```python
from build123d import *

# Parameters (mm, degrees)
SKETCH1_R           = 2.3
SKETCH1_R_2         = 4
BOSS_EXTRUDE1_DEPTH = 22.25
FILLET1_R           = 1
FILLET2_R           = 0.5


with BuildPart() as part:
    # Sketch1 → Boss-Extrude1 (new body)
    # profile 1 of 4: a face of its own
    with BuildSketch(Plane(origin=(0, 0, 0), x_dir=(1, 0, 0), z_dir=(0, 1, 0))):
        with BuildLine():
            ThreePointArc((4, 25.4), (0, 21.4), (-4, 25.4))
            Line((-4, 25.4), (-4, 0))
            ThreePointArc((-4, 0), (0, 4), (4, 0))
            ThreePointArc((4, 0), (3.526698395, -1.887431702), (2.218800785, -3.328201177))
            Line((2.218800785, -3.328201177), (40.318800785, 22.071798823))
            ThreePointArc((40.318800785, 22.071798823), (34.271631894, 24.240863405), (38.1, 29.4))
            Line((38.1, 29.4), (0, 29.4))
            ThreePointArc((0, 29.4), (2.828427125, 28.228427125), (4, 25.4))
        make_face()
        Polygon((4, 5.070367517), (4, 21.4), (28.494448725, 21.4), align=None, mode=Mode.SUBTRACT)
        with Locations(Location((12.7, 25.4, 0), (0, 0, 270))):
            Circle(SKETCH1_R, mode=Mode.SUBTRACT)
    # profile 2 of 4: a face of its own
    with BuildSketch(Plane(origin=(0, 0, 0), x_dir=(1, 0, 0), z_dir=(0, 1, 0))):
        Circle(SKETCH1_R_2)
        with Locations(Location((0, 0, 0), (0, 0, 270))):
            Circle(SKETCH1_R, mode=Mode.SUBTRACT)
    # profile 3 of 4: a face of its own
    with BuildSketch(Plane(origin=(0, 0, 0), x_dir=(1, 0, 0), z_dir=(0, 1, 0))):
        with Locations((38.1, 25.4)):
            Circle(SKETCH1_R_2)
        with Locations(Location((38.1, 25.4, 0), (0, 0, 270))):
            Circle(SKETCH1_R, mode=Mode.SUBTRACT)
    # profile 4 of 4: a face of its own
    with BuildSketch(Plane(origin=(0, 0, 0), x_dir=(1, 0, 0), z_dir=(0, 1, 0))):
        with Locations((0, 25.4)):
            Circle(SKETCH1_R_2)
        with Locations(Location((0, 25.4, 0), (0, 0, 270))):
            Circle(SKETCH1_R, mode=Mode.SUBTRACT)
    extrude(amount=BOSS_EXTRUDE1_DEPTH)

    # Fillet1
    fillet1_edges = [part.edges().sort_by_distance(p)[0] for p in [
        (4, 11.125, -21.4),
        (4, 11.125, -5.070367517),
        (28.494448725, 11.125, -21.4),
    ]]
    fillet(fillet1_edges, radius=FILLET1_R)

    # Fillet2
    fillet2_edges = [part.edges().sort_by_distance(p)[0] for p in [
        (19.05, 22.25, -29.4),
        (-2.828427125, 22.25, -28.228427125),
        (41.928368106, 0, -26.559136595),
        (21.268800785, 0, -9.371798823),
        (-4, 22.25, -12.7),
        (-1.887431702, 0, 3.526698395),
        (-4, 0, -12.7),
        (-2.828427125, 0, -28.228427125),
        (19.05, 0, -29.4),
        (-1.887431702, 22.25, 3.526698395),
        (21.268800785, 22.25, -9.371798823),
        (41.928368106, 22.25, -26.559136595),
        (15.65053674, 0, -12.83739201),
        (15.65053674, 22.25, -12.83739201),
        (15.095836543, 0, -21.4),
        (15.095836543, 22.25, -21.4),
        (4, 0, -13.669442304),
        (4, 22.25, -13.669442304),
        (26.148765113, 0, -20.689784149),
        (26.148765113, 22.25, -20.689784149),
        (4.528142074, 0, -6.05721001),
        (4.528142074, 22.25, -6.05721001),
        (4.292893219, 0, -21.107106781),
        (4.292893219, 22.25, -21.107106781),
    ]]
    fillet(fillet2_edges, radius=FILLET2_R)


solid = part.part
```
The model under review builds one solid part; all positions refer to its coordinate system, in mm. A direction names the side the tool comes from. Round coordinates to 2 decimals unless told otherwise and drop trailing zeros. Write each loop counter-clockwise with the first axis right and the second up, starting at its lowest first coordinate (ties: lowest second). Pieces come first, ordered by that corner, then holes.
(1) We need section A-A on y = 10.75. Give the boundary of the cut face in (x, z), and give its area (3 significant figures).
(2) We need section B-B on x = 12.7. Give the number of separate pieces and of enclosed holes in the cut face, and give its area (3 significant figures).
(3) Machinability: for faces 5 (the cylindrical face through (4.301, 11.274, -21.115)), 6 (the cylindrical face through (15.588, 0.15, -12.625)), 7 (the flat face through (-4, 11, -13)), which of the approach directions +Z, -Z, +X, -X, +Y, -Y give a long, thin tool a straight path to every point of the face, cutting with its end or side? Answer none if there is none.
(4) Wall thickness on L1, parallel to X at y = 17.25, z = -25.4; L2, parallel to Z at x = -1.5, y = 11.25; L3, parallel to Z at x = 13.5, y = 13: over which ranges is each line inside the solid? List them lowest first.
(5) Insertion check: pin 1 (6 mm diameter, centred on x = 34.5, y = 14.5, fed in from +Z); pin 2 (8 mm diameter, centred on x = 34, z = -15.5, fed in from -Y); pin 3 (3 mm diameter, centred on x = 38.1, z = -25.4, fed in from +Y); pin 4 (1 mm diameter, centred on x = 37, y = 5, fed in from +Z). Each pin has a flat end and moves straight along its axis. Give the tip position at first contact, or say it passes through.
(6) Mouldability with a two-part tool opening along Z and no side actions: class faces 1 (the cylindrical face through (26.154, 11.274, -20.673)), 2 (the flat face through (15.79, 10.98, -12.93)), 3 (the flat face through (19, 22.25, -13)), 4 (the cylindrical face through (-1.94, 10.98, 3.5)) as +Z half, -Z half, draft (parallel to the pull), parting line (faces both ways), or undercut.
Findings below:
1. outline: (-4, -25.4) arc R4 ccw to (0, -29.4) - (38.1, -29.4) arc R4 ccw to (40.32, -22.07) - (2.22, 3.33) arc R4 ccw to (-4, 0) - close; hole circle Ø4.6 at (0, -25.4); hole circle Ø4.6 at (0, 0); hole (4, -20.4) arc R1 ccw to (5, -21.4) - (25.19, -21.4) arc R1 ccw to (25.75, -19.57) - (5.55, -6.11) arc R1 ccw to (4, -6.94) - close; hole circle Ø4.6 at (12.7, -25.4); hole circle Ø4.6 at (38.1, -25.4)
1. area: 708 mm2
2. separate pieces: 3
2. enclosed holes: 0
2. area: 236 mm2
3. face 5: +Y, -Y
3. face 6: -Y
3. face 7: +Z, -Z, -X, +Y, -Y
4. L1: x = -4 to -2.3, 2.3 to 10.4, 15 to 35.8, 40.4 to 42.1
4. L2: z = -29.11 to -27.14, -23.66 to -1.74, 1.74 to 3.71
4. L3: z = -29.4 to -27.56, -23.24 to -21.4, -11.4 to -4.19
5. pin 1: stops at z = -16.19
5. pin 2: stops at y = 0
5. pin 3: passes through
5. pin 4: stops at z = -19.53
6. face 1: undercut
6. face 2: undercut
6. face 3: draft
6. face 4: +Z half
